from build123d import *

# Parameters (mm, degrees)
SKETCH1_W           = 256
SKETCH1_H           = 50
SKETCH1_R           = 2
BOSS_EXTRUDE1_DEPTH = 8
FILLET1_R           = 4
SKETCH2_W           = 7
SKETCH2_H           = 8
BOSS_EXTRUDE2_DEPTH = 8
SKETCH3_W           = 50
SKETCH3_H           = 20
CUT_EXTRUDE1_DEPTH  = 8
SKETCH4_R           = 2
CUT_EXTRUDE2_DEPTH  = 8
SKETCH5_R           = 1.75
CUT_EXTRUDE3_DEPTH  = 113


with BuildPart() as part:
    # Sketch1 → Boss-Extrude1 (new body)
    with BuildSketch(Plane.XY):
        with Locations((0.283809042, 47.106089777)):
            Rectangle(SKETCH1_W, SKETCH1_H)
        with Locations((120.283809042, 65.106089777)):
            Circle(SKETCH1_R, mode=Mode.SUBTRACT)
        with Locations((111.283809042, 65.106089777)):
            Circle(SKETCH1_R, mode=Mode.SUBTRACT)
        with Locations((8.283809042, 65.106089777)):
            Circle(SKETCH1_R, mode=Mode.SUBTRACT)
        with Locations((-7.716190958, 65.106089777)):
            Circle(SKETCH1_R, mode=Mode.SUBTRACT)
        with Locations((-16.716190958, 65.106089777)):
            Circle(SKETCH1_R, mode=Mode.SUBTRACT)
        with Locations((-119.716190958, 65.106089777)):
            Circle(SKETCH1_R, mode=Mode.SUBTRACT)
    extrude(amount=BOSS_EXTRUDE1_DEPTH)

    # Fillet1
    fillet1_edges = [part.edges().sort_by_distance(p)[0] for p in [
        (-127.716190958, 72.106089777, 4),
        (128.283809042, 72.106089777, 4),
        (128.283809042, 22.106089777, 4),
        (-127.716190958, 22.106089777, 4),
    ]]
    fillet(fillet1_edges, radius=FILLET1_R)

    # Sketch2 → Boss-Extrude2 (add)
    with BuildSketch(Plane.XY.offset(8)):
        with Locations((36.783809042, 18.106089777)):
            Rectangle(SKETCH2_W, SKETCH2_H)
        with Locations((-36.216190958, 18.106089777)):
            Rectangle(SKETCH2_W, SKETCH2_H)
    extrude(amount=-BOSS_EXTRUDE2_DEPTH)

    # Sketch3 → Cut-Extrude1 (cut)
    with BuildSketch(Plane.XY.offset(8)):
        with Locations((0.283809042, 32.106089777)):
            Rectangle(SKETCH3_W, SKETCH3_H)
    extrude(amount=-CUT_EXTRUDE1_DEPTH, mode=Mode.SUBTRACT)

    # Sketch4 → Cut-Extrude2 (cut)
    with BuildSketch(Plane.XY.offset(8)):
        with Locations((-31.716190958, 32.106089777)):
            Circle(SKETCH4_R)
        with Locations((32.283809042, 32.106089777)):
            Circle(SKETCH4_R)
        with Locations((-119.716190958, 32.106089777)):
            Circle(SKETCH4_R)
        with Locations((120.283809042, 29.106089777)):
            Circle(SKETCH4_R)
    extrude(amount=-CUT_EXTRUDE2_DEPTH, mode=Mode.SUBTRACT)

    # Sketch5 → Cut-Extrude3 (cut)
    with BuildSketch(Plane.ZY.offset(39.716190958)):
        with Locations((3.5, 18.106089777)):
            Circle(SKETCH5_R)
    extrude(amount=-CUT_EXTRUDE3_DEPTH, mode=Mode.SUBTRACT)


solid = part.part
Geometry check sheet. Reference: the model listing, model coordinates, mm. A direction names the side the tool comes from. Round coordinates to 2 decimals unless told otherwise and drop trailing zeros. Write each loop counter-clockwise with the first axis right and the second up, starting at its lowest first coordinate (ties: lowest second). Pieces come first, ordered by that corner, then holes.
Item 1: Material ranges on line 1 along X through (y, z) = (31.5, 7.75); line 2 along Y through (x, z) = (35, 3.5); line 3 along X through (y, z) = (33.5, 6.25), recorded low to high.
Determined:
line 1: x = -127.72 to -121.62, -117.81 to -33.62, -29.81 to -24.72, 25.28 to 30.38, 34.19 to 128.28
line 2: y = 14.11 to 16.36, 19.86 to 72.11
line 3: x = -127.72 to -121.15, -118.28 to -33.15, -30.28 to -24.72, 25.28 to 30.85, 33.72 to 128.28
Item 2: Section check B-B (z = 3.5). Give the number of separate pieces and of enclosed holes in the cut face, plus the area to 3 significant figures.
Determined:
separate pieces: 3
enclosed holes: 10
area: 11,700 mm2
Item 3: Section check A-A (y = 38). Record the boundary of the cut face in (x, z), plus the area to 3 significant figures.
Determined:
outline: (-127.72, 0) - (-24.72, 0) - (-24.72, 8) - (-127.72, 8) - close; (25.28, 0) - (128.28, 0) - (128.28, 8) - (25.28, 8) - close
area: 1,650 mm2
Item 4: Section check D-D (x = 81.5). Record the boundary of the cut face in (y, z), plus the area to 3 significant figures.
Determined:
outline: (22.11, 0) - (72.11, 0) - (72.11, 8) - (22.11, 8) - close
area: 400 mm2
Item 5: Access from +Z, -Z, +X, -X, +Y, -Y to the whole of each face (thin tool, end or side, straight path). Record for faces 4 (the face through (40.284, 18, 6)), 5 (the face through (-39.716, 18, 6)), 6 (the face through (-24.716, 32, 4)), 7 (the face through (-1, 72.106, 4)), 8 (the face through (-126.58, 70.9, 4.06)).
Determined:
face 4: +Z, -Z, +X, -Y
face 5: +Z, -Z, -X, -Y
face 6: +Z, -Z, -Y
face 7: +Z, -Z, +X, -X, +Y
face 8: +Z, -Z, -X, +Y
Item 6: Mould release check, pull along Y, two halves, no side actions. Record for faces 1 (the face through (-8.15, 63.154, 3.944)), 2 (the face through (0, 42.106, 4)), 3 (the face through (127.081, 70.965, 4.056)): +Y half, -Y half, draft (parallel to the pull), parting line (faces both ways), or undercut.
Determined:
face 1: undercut
face 2: -Y half
face 3: +Y half
Item 7: Go/stop test with flat-tipped pins: pin 1 Ø2.5 at (x, y) = (32.28, 32.11) entering from +Z; pin 2 Ø2.5 at (x, z) = (-82.5, 2) entering from -Y. Record where each tip stops, or that it passes through.
Determined:
pin 1: passes through
pin 2: stops at y = 22.11
Item 8: Section check C-C (x = 17). Record the boundary of the cut face in (y, z).
Determined:
outline: (42.11, 0) - (72.11, 0) - (72.11, 8) - (42.11, 8) - close
